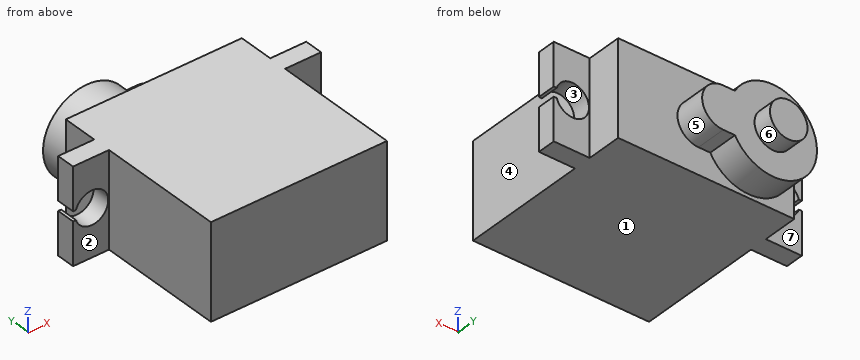
from build123d import *

# Parameters (mm, degrees)
BOSS_EXTRUDE1_DEPTH = 6.175
BOSS_EXTRUDE2_DEPTH = 4
SKETCH4_R           = 2.45
BOSS_EXTRUDE3_DEPTH = 2.5
CUT_EXTRUDE1_REACH  = 36.097


with BuildPart() as part:
    # Sketch1 → Boss-Extrude1 (new, symmetric)
    with BuildSketch(Plane.XY):
        Polygon((0, 0), (23, 0), (23, 16.5), (27.7, 16.5), (27.7, 18.9), (23, 18.9), (23, 23.5), (0, 23.5), (0, 18.9), (-4.7, 18.9), (-4.7, 16.5), (0, 16.5), align=None)
    extrude(amount=BOSS_EXTRUDE1_DEPTH, both=True)

    # Sketch3 → Boss-Extrude2 (add)
    with BuildSketch(Plane(origin=(0, 23.5, 0), x_dir=(1, 0, 0), z_dir=(0, 1, 0))):
        with BuildLine():
            Line((12.5, 2.75), (10.964158271, 2.75))
            ThreePointArc((10.964158271, 2.75), (0.25, 0), (10.964158271, -2.75))
            Line((10.964158271, -2.75), (12.5, -2.75))
            ThreePointArc((12.5, -2.75), (15.25, 0), (12.5, 2.75))
        make_face()
    extrude(amount=BOSS_EXTRUDE2_DEPTH)

    # Sketch4 → Boss-Extrude3 (add)
    with BuildSketch(Plane(origin=(0, 27.5, 0), x_dir=(1, 0, 0), z_dir=(0, 1, 0))):
        with Locations(Location((5.96, 0, 0), (0, 0, 180))):
            Circle(SKETCH4_R)
    extrude(amount=BOSS_EXTRUDE3_DEPTH)

    # Sketch5 → Cut-Extrude1 (cut, up to next)
    with BuildSketch(Plane(origin=(0, 18.9, 0), x_dir=(1, 0, 0), z_dir=(0, 1, 0)), mode=Mode.PRIVATE) as cut_extrude1_sk1:
        with BuildLine():
            Line((-4.7, 0.625), (-4.311332336, 0.625))
            ThreePointArc((-4.311332336, 0.625), (-0.096, 0), (-4.311332336, -0.625))
            Line((-4.311332336, -0.625), (-4.7, -0.625))
            Line((-4.7, -0.625), (-4.7, 0.625))
        make_face()
    cut_extrude1_tool1 = extrude(cut_extrude1_sk1.sketch, amount=-CUT_EXTRUDE1_REACH, mode=Mode.PRIVATE) & part.part
    # Sketch5 → Cut-Extrude1 (cut, up to next)
    with BuildSketch(Plane(origin=(0, 18.9, 0), x_dir=(1, 0, 0), z_dir=(0, 1, 0)), mode=Mode.PRIVATE) as cut_extrude1_sk2:
        with BuildLine():
            Line((27.311332336, 0.625), (27.7, 0.625))
            Line((27.7, 0.625), (27.7, -0.625))
            Line((27.7, -0.625), (27.311332336, -0.625))
            ThreePointArc((27.311332336, -0.625), (23.096, 0), (27.311332336, 0.625))
        make_face()
    cut_extrude1_tool2 = extrude(cut_extrude1_sk2.sketch, amount=-CUT_EXTRUDE1_REACH, mode=Mode.PRIVATE) & part.part
    add(cut_extrude1_tool1.solids().sort_by_distance((-2.312273, 18.9, 0))[0], mode=Mode.SUBTRACT)
    add(cut_extrude1_tool2.solids().sort_by_distance((25.312273, 18.9, 0))[0], mode=Mode.SUBTRACT)


solid = part.part
Build history of the part. All positions in model axes, mm. Face numbers are marked on the shaded views. A direction names the side the tool comes from. Give positions to 0.01 mm unless a question says otherwise; leave off trailing zeros. Order: outer loops, then holes, each group sorted by start corner. A loop starts at its lowest first (then second) coordinate and runs counter-clockwise, first axis right, second up. Notation, with made-up numbers: M 76,37.25 L 103,37.25 A20 ccw 103,72.25 Z; hole C 4,-18.5 d5. An arc over 180 degrees is marked long. Put each result on its own line as item: value.
Item 1: Which spindle directions (+Z, -Z, +X, -X, +Y, -Y) get a long thin tool onto all of the face, cutting with end or side? Do the marked faces 4, 5, 6 and 7. Say none if no direction does.
Results are:
face 4: +Z, -Z, +X, -Y
face 5: +X, +Y
face 6: +Y
face 7: +Z, -Z, -X, +Y
Item 2: Cut at A-A on x = 25.25. Write the cut outline in (y, z) (3 decimals), then the cut area to 3 significant figures.
Results are:
outline: M 16.5,-6.175 L 18.9,-6.175 L 18.9,-2.154 L 16.5,-2.154 Z; M 16.5,2.154 L 18.9,2.154 L 18.9,6.175 L 16.5,6.175 Z
area: 19.3 mm2
Item 3: Pull direction Z, two halves, no side cores. Call the marked faces 1, 2 and 3: +Z half, -Z half, draft (parallel to the pull), parting line (faces both ways), or undercut.
Results are:
face 1: -Z half
face 2: draft
face 3: undercut
Item 4: Cut at D-D on z = -4.75. Write the cut outline in (x, y).
Results are:
outline: M -4.7,16.5 L 0,16.5 L 0,0 L 23,0 L 23,16.5 L 27.7,16.5 L 27.7,18.9 L 23,18.9 L 23,23.5 L 9.13,23.5 L 9.13,27.5 L 2.79,27.5 L 2.79,23.5 L 0,23.5 L 0,18.9 L -4.7,18.9 Z
Item 5: Cut at B-B on z = 1. Write the cut outline in (x, y), then the cut area to 3 significant figures.
Results are:
outline: M -4.7,16.5 L -4.16,16.5 L -4.16,18.9 L -4.7,18.9 Z; M -0.34,16.5 L 0,16.5 L 0,0 L 23,0 L 23,16.5 L 23.34,16.5 L 23.34,18.9 L 23,18.9 L 23,23.5 L 15.06,23.5 L 15.06,27.5 L 8.2,27.5 L 8.2,30 L 3.72,30 L 3.72,27.5 L 0.34,27.5 L 0.34,23.5 L 0,23.5 L 0,18.9 L -0.34,18.9 Z; M 27.16,16.5 L 27.7,16.5 L 27.7,18.9 L 27.16,18.9 Z
area: 615 mm2
Item 6: Drop flat-ended pins along their axis: pin 1 Ø1.4 at (y, z) = (22, 2.5) entering from -X; pin 2 Ø4 at (x, y) = (23.5, 26.5) entering from -Z; pin 3 Ø3.5 at (y, z) = (21, 3) entering from +X; pin 4 Ø1.7 at (x, y) = (11.5, 24.5) entering from -Z. Give the stop position or say it passes through.
Results are:
pin 1: x = 0
pin 2: through
pin 3: x = 23
pin 4: z = -3.26
Item 7: Wall check: probe 1 along Z at (x, y) = (25.25, 17.35) (3 decimals); probe 2 along X at (y, z) = (17.3, 0); probe 3 along Y at (x, z) = (14, 4.5). Give the ranges that are in metal, low to high.
Results are:
probe 1: -6.175 to -2.154, 2.154 to 6.175
probe 2: -0.1 to 23.1
probe 3: 0 to 23.5
Item 8: Cut at C-C on x = 5.96. Write the cut outline in (y, z) (3 decimals).
Results are:
outline: M 0,-6.175 L 23.5,-6.175 L 23.5,-5.71 L 27.5,-5.71 L 27.5,-2.45 L 30,-2.45 L 30,2.45 L 27.5,2.45 L 27.5,5.71 L 23.5,5.71 L 23.5,6.175 L 0,6.175 Z
